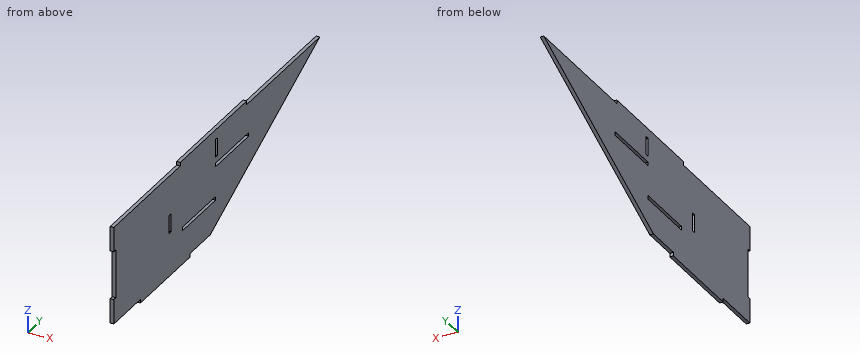
from build123d import *

# Parameters (mm, degrees)
SALIENTE_EXTRUIR1_DEPTH = 3
CROQUIS2_W              = 3
CROQUIS2_H              = 50
CORTAR_EXTRUIR2_DEPTH   = 70
CROQUIS4_W              = 15
CROQUIS4_H              = 3
CORTAR_EXTRUIR3_DEPTH   = 3


with BuildPart() as part:
    # Croquis1 → Saliente-Extruir1 (new body)
    with BuildSketch(Plane(origin=(0, 0, 0), x_dir=(0, 0, -1), z_dir=(1, 0, 0))):
        Polygon((0, 0), (0, 100), (-3, 100), (-3, 200), (0, 200), (0, 310), (81, 145), (81, 115), (84, 115), (84, 40), (81, 40), (81, 0), (60.5, 0), (60.5, 3), (20.5, 3), (20.5, 0), align=None)
    extrude(amount=SALIENTE_EXTRUIR1_DEPTH)

    # Croquis2 → Cortar-Extruir2 (cut)
    with BuildSketch(Plane(origin=(3, 0, 0), x_dir=(0, 0, -1), z_dir=(1, 0, 0))):
        with Locations((26.5, 178)):
            Rectangle(CROQUIS2_W, CROQUIS2_H)
        with Locations((54.5, 128)):
            Rectangle(CROQUIS2_W, CROQUIS2_H)
    extrude(amount=-CORTAR_EXTRUIR2_DEPTH, mode=Mode.SUBTRACT)

    # Croquis4 → Cortar-Extruir3 (cut)
    with BuildSketch(Plane(origin=(3, 0, 0), x_dir=(0, 0, -1), z_dir=(1, 0, 0))):
        with Locations((12.5, 154.5)):
            Rectangle(CROQUIS4_W, CROQUIS4_H)
        with Locations((40.5, 84.5)):
            Rectangle(CROQUIS4_W, CROQUIS4_H)
    extrude(amount=-CORTAR_EXTRUIR3_DEPTH, mode=Mode.SUBTRACT)


solid = part.part
Geometry check sheet. Reference: the model listing, model coordinates, mm. Coordinates: 2 decimals unless noted, no trailing zeros. Order: outer loops, then holes, each group sorted by start corner. A loop starts at its lowest first (then second) coordinate and runs counter-clockwise, first axis right, second up. Notation, with made-up numbers: (63.5, 83) -> (104.5, 83) arc R27 ccw to (104.5, 112) -> close; hole circle Ø11 at (-29.5, 46.25). An arc over 180 degrees is marked (long way). Use a Markdown table: item, result. Add a question column.
1. Cross-section at D-D (y = 22). Enter the section's corners in (x, z), and give its area (3 significant figures).
2. Go/stop test with flat-tipped pins: pin 1 Ø1.5 at (x, y) = (1, 84) entering from +Z; pin 2 Ø0.9 at (x, z) = (1.5, -13) entering from +Y; pin 3 Ø1.5 at (x, y) = (1, 137) entering from -Z. Record where each tip stops, or that it passes through.
3. Cross-section at B-B (y = 179). Enter the section's corners in (x, z).
4. Cross-section at C-C (z = -15). Enter the section's corners in (x, y).
5. Material ranges on L1, parallel to Z at x = 1.5, y = 136; L2, parallel to Y at x = 0.5, z = -34; L3, parallel to Y at x = 2, z = -43.5, recorded low to high.
6. Cross-section at A-A (x = 2.2). Give the number of separate pieces and of enclosed holes in the cut face, and give its area (3 significant figures).
Filled sheet:
| question | item | result |
|---|---|---|
| 1 | outline | (0, -81) -> (3, -81) -> (3, 0) -> (0, 0) -> close |
| 1 | area | 243 mm2 |
| 2 | pin 1 | z = 0 |
| 2 | pin 2 | y = 284.44 |
| 2 | pin 3 | z = -81 |
| 3 | outline | (0, -64.31) -> (3, -64.31) -> (3, -28) -> (0, -28) -> close; (0, -25) -> (3, -25) -> (3, 3) -> (0, 3) -> close |
| 4 | outline | (0, 0) -> (3, 0) -> (3, 153) -> (0, 153) -> close; (0, 156) -> (3, 156) -> (3, 279.44) -> (0, 279.44) -> close |
| 5 | L1 | -81 to -56, -53 to 3 |
| 5 | L2 | 3 to 83, 86 to 240.74 |
| 5 | L3 | 3 to 83, 86 to 221.39 |
| 6 | separate pieces | 1 |
| 6 | enclosed holes | 4 |
| 6 | area | 18,400 mm2 |
